The model under review builds one solid part; all positions refer to its coordinate system, in mm. Face numbers are marked on the shaded views. Round coordinates to 2 decimals unless told otherwise and drop trailing zeros. Loops run counter-clockwise (first coordinate to the right, second up) from the corner with the lowest first, then second, coordinate; pieces in that order, holes last. Notation, with made-up numbers: M 16.25,37.25 L 73.25,37.25 A19 ccw 73.25,73.25 Z; hole C 45,-32 d9. An arc over 180 degrees is marked long. Return JSON: item names as keys, results as strings. Group by question number.
Q1. Consider section A-A (z = 0). State the section outline as (x, y) points (3 decimals), and give its area (3 significant figures).
Q2. Clearance check with a flat-ended pin moving along its axis: pin 1 Ø1.5 at (y, z) = (1.5, -1) entering from -X. State where the tip first meets the part, or that it passes through.
Q3. To check wall thickness, follow line 1 along Y through (x, z) = (-0.65, 0) (3 decimals); line 2 along Z through (x, y) = (-1.1, 3.75); line 3 along Y through (x, z) = (1.65, -0.6). State the ranges of each line that lie inside material, in increasing order.
Q4. Consider section C-C (y = 3.5). State the section outline as (x, z) points.
Q5. Consider section B-B (x = 0). State the section outline as (y, z) points (3 decimals).
Q6. Draft analysis for pull direction Y (two halves, no side actions). For the marked faces 1, 2 and 3, state which applies: pulls with the +Y half, pulls with the -Y half, needs draft (parallel to the pull), parting line crosses it, or undercut.
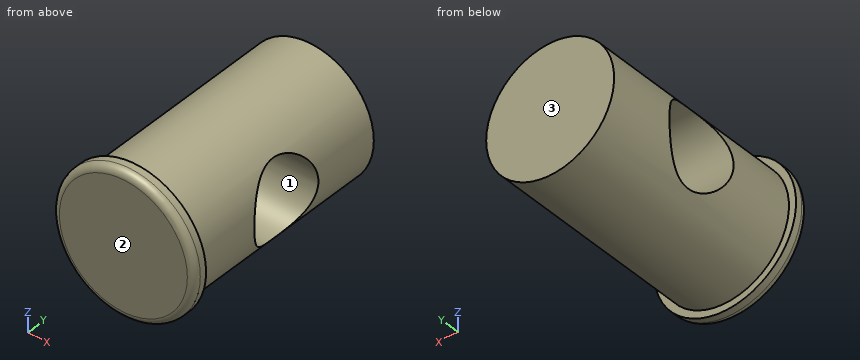
from build123d import *

# Parameters (mm, degrees)
F0_R     = 2.286
F1_DEPTH = 8.128
F0_R_2   = 2.54
F2_DEPTH = 0.508
F3_R     = 1.397
F4_DEPTH = 12.7
F5_R     = 0.254


with BuildPart() as f1:
    # F0 (on Front) → F1 (new body)
    with BuildSketch(Plane.XZ):
        Circle(F0_R)
    extrude(amount=-F1_DEPTH)

    # F0 (on Front) → F2 (join)
    with BuildSketch(Plane.XZ):
        Circle(F0_R_2)
        Circle(F0_R, mode=Mode.SUBTRACT)
    extrude(amount=-F2_DEPTH)

    # F3 (on Right) → F4 (cut, symmetric)
    with BuildSketch(Plane.YZ):
        with Locations((4.318, 0)):
            Circle(F3_R)
    extrude(amount=F4_DEPTH, both=True, mode=Mode.SUBTRACT)

    # F5
    f5_edges = [f1.edges().sort_by_distance(p)[0] for p in [
        (-2.54, 0, 0),
    ]]
    fillet(f5_edges, radius=F5_R)


solid = f1.part
Values:
{
 "1": {"outline": "M -2.54,0.254 A0.254 ccw -2.286,0 L 2.286,0 A0.254 ccw 2.54,0.254 L 2.54,0.508 L 2.286,0.508 L 2.286,2.921 L -2.286,2.921 L -2.286,0.508 L -2.54,0.508 Z; M -2.286,5.715 L 2.286,5.715 L 2.286,8.128 L -2.286,8.128 Z", "area": "24.6 mm2"},
 "2": {"pin 1": "stops at x = -2.27"},
 "3": {"line 1": "y = 0 to 2.921, 5.715 to 8.128", "line 2": "z = -2 to -1.28, 1.28 to 2", "line 3": "y = 0 to 3.06, 5.58 to 8.13"},
 "4": {"outline": "M -1.99,-1.13 A2.29 ccw 1.99,-1.13 Z; M -1.99,1.13 L 1.99,1.13 A2.29 ccw Z"},
 "5": {"outline": "M 0,-2.286 A0.254 ccw 0.254,-2.54 L 0.508,-2.54 L 0.508,-2.286 L 8.128,-2.286 L 8.128,2.286 L 0.508,2.286 L 0.508,2.54 L 0.254,2.54 A0.254 ccw 0,2.286 Z; hole C 4.318,0 d2.794"},
 "6": {"face 1": "undercut", "face 2": "pulls with the -Y half", "face 3": "pulls with the +Y half"}
}
